Geometry: see drawing. Coordinates: mm, zero at the bounding-box minimum. Give positions to 0.01 mm unless a question says otherwise; leave off trailing zeros. Order: outer loops, then holes, each group sorted by start corner. A loop starts at its lowest first (then second) coordinate and runs counter-clockwise, first axis right, second up. Notation, with made-up numbers: (12, 51.25) - (58, 51.25) arc R25 cw to (58, 68.25) - close; hole circle Ø7 at (34.25, -2). An arc over 180 degrees is marked (long way). Write each question's results on one line, items separated by ' | '. Start each with the question number.
Item 1: Section A-A on x = 2. Output: boundary loops of the cut face in (y, z).
Item 2: Line query: line 1 along Z through (x, y) = (0.5, 4.5) (1 decimal); line 2 along Z through (x, y) = (2.05, 3.75) (1 decimal); line 3 along Y through (x, z) = (1.4, 6.5) (1 decimal). Output: solid intervals per line, ascending.
Item 3: Mould query, pull axis Y, two halves, no side actions, for the marked faces 1, 2 and 3. Classes: released by +Y, released by -Y, zero draft, split by the parting line, or undercut.
Item 4: Section B-B on x = 3.05. Output: boundary loops of the cut face in (y, z), and give its area (3 significant figures).
Item 5: Contact query for a flat-ended pin moving along its axis: pin 1 Ø1 at (x, z) = (2.5, 8) entering from +Y (1 decimal). Output: stop coordinate, or through.
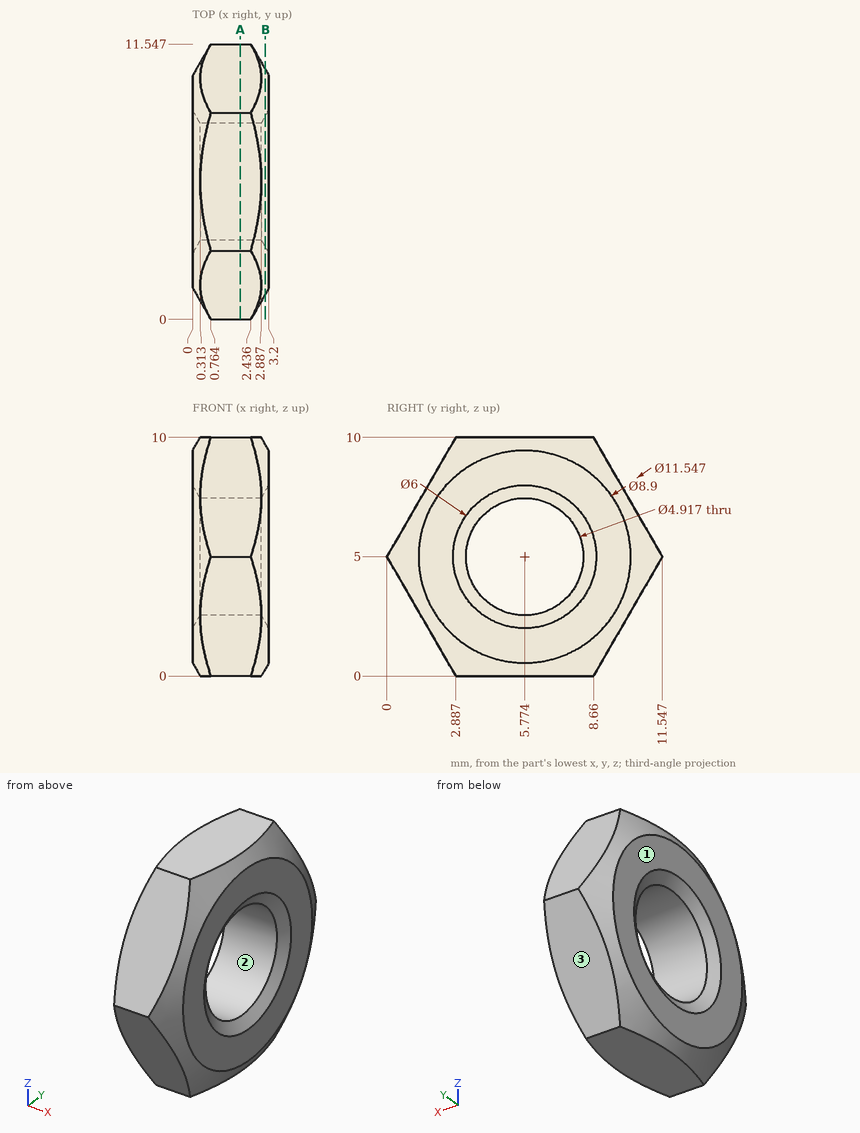
Evaluation:
1) outline: (0, 5) - (2.89, 0) - (8.66, 0) - (11.55, 5) - (8.66, 10) - (2.89, 10) - close; hole circle Ø4.92 at (5.77, 5)
2) line 1: z = 0 to 2.9, 7.1 to 10 | line 2: z = 0 to 3.6, 6.4 to 10 | line 3: y = 0.9 to 3.8, 7.7 to 10.7
3) face 1: zero draft | face 2: undercut | face 3: released by +Y
4) outline: circle Ø9.42 at (5.77, 5); hole circle Ø5.48 at (5.77, 5) | area: 46.1 mm^2
5) pin 1: stops at y = 10.1
